Input: part model. Units: mm. Frame: model coordinates. Coordinates: 2 decimals unless noted, no trailing zeros. Write each loop counter-clockwise with the first axis right and the second up, starting at its lowest first coordinate (ties: lowest second). Pieces come first, ordered by that corner, then holes.
1) Pin query (flat end, axial travel): pin 1 Ø1.4 at (x, z) = (30, 3.5) entering from +Y; pin 2 Ø1.4 at (x, z) = (27, 1.5) entering from -Y; pin 3 Ø2 at (y, z) = (56.5, 1.5) entering from +X. Return the tip coordinate at first contact, or that it passes through.
2) Draft query along X for faces 1 (the flat face through (40.2, 62.9, 2.3)), 2 (the flat face through (53, 38, 4.572)). Return one class per face: pulls with the +X half, pulls with the -X half, needs draft (parallel to the pull), parting line crosses it, or undercut.
3) Section query C-C (z = 2.65). State how many separate pieces and enclosed holes the cut face has, then the cut area to 3 significant figures.
4) Line query: L1, parallel to Y at x = -2.5, z = 0.4 (1 decimal); L2, parallel to Y at x = 65.5, z = 3.2; L3, parallel to X at y = 42.5, z = 1. Output: solid intervals per line, ascending.
5) Section query A-A (y = 46). Output: boundary loops of the cut face in (x, z), then the cut area to 3 significant figures.
6) Section query B-B (x = 91). Output: boundary loops of the cut face in (y, z), then the cut area to 3 significant figures.
from build123d import *

# Parameters (mm, degrees)
SKETCH1_R           = 2.5527
SKETCH1_R_2         = 4.1275
SKETCH1_R_3         = 19.177
BOSS_EXTRUDE1_DEPTH = 4.572


with BuildPart() as part:
    # Sketch1 → Boss-Extrude1 (new body)
    with BuildSketch(Plane.XY):
        with BuildLine():
            Line((-17.186005785, 5.917481167), (-17.186005785, 69.562080021))
            ThreePointArc((-17.186005785, 69.562080021), (-15.770600509, 73.558612882), (-12.155368019, 75.773503633))
            Line((-12.155368019, 75.773503633), (114.857780393, 75.773503633))
            ThreePointArc((114.857780393, 75.773503633), (119.939137204, 73.478410267), (121.251078966, 68.059328295))
            Line((121.251078966, 68.059328295), (121.251078966, 4.414729441))
            ThreePointArc((121.251078966, 4.414729441), (118.772241914, 0.732566989), (114.487440215, -0.426496367))
            Line((114.487440215, -0.426496367), (-11.1125, -0.426496367))
            ThreePointArc((-11.1125, -0.426496367), (-15.422847741, 1.526196519), (-17.186005785, 5.917481167))
        make_face()
        with Locations((90.763994215, 5.917481167)):
            Circle(SKETCH1_R, mode=Mode.SUBTRACT)
        with Locations((90.763994215, 69.562080021)):
            Circle(SKETCH1_R, mode=Mode.SUBTRACT)
        with Locations((-10.836005785, 69.562080021)):
            Circle(SKETCH1_R, mode=Mode.SUBTRACT)
        with Locations((39.963994215, 69.562080021)):
            Circle(SKETCH1_R, mode=Mode.SUBTRACT)
        with Locations((-10.836005785, 5.917481167)):
            Circle(SKETCH1_R, mode=Mode.SUBTRACT)
        with Locations((39.963994215, 5.917481167)):
            Circle(SKETCH1_R, mode=Mode.SUBTRACT)
        with Locations((63.001987758, 56.151789166)):
            Circle(SKETCH1_R_2, mode=Mode.SUBTRACT)
        with Locations((115.233146458, 39.581556975)):
            Circle(SKETCH1_R, mode=Mode.SUBTRACT)
        with Locations((98.923012242, 20.230764682)):
            Circle(SKETCH1_R_2, mode=Mode.SUBTRACT)
        with Locations((80.9625, 38.1)):
            Circle(SKETCH1_R_3, mode=Mode.SUBTRACT)
        Polygon((1.103378735, 60.325), (-1.829560633, 65.405), (-7.695439367, 65.405), (-10.628378735, 60.325), (-7.695439367, 55.245), (-1.829560633, 55.245), align=None, mode=Mode.SUBTRACT)
        Polygon((50.443227049, 60.325), (47.510287682, 65.405), (41.644408947, 65.405), (38.71146958, 60.325), (41.644408947, 55.245), (47.510287682, 55.245), align=None, mode=Mode.SUBTRACT)
        Polygon((1.103378735, 16.331279268), (-1.829560633, 21.411279268), (-7.695439367, 21.411279268), (-10.628378735, 16.331279268), (-7.695439367, 11.251279268), (-1.829560633, 11.251279268), align=None, mode=Mode.SUBTRACT)
        Polygon((50.443227049, 16.331279268), (47.510287682, 21.411279268), (41.644408947, 21.411279268), (38.71146958, 16.331279268), (41.644408947, 11.251279268), (47.510287682, 11.251279268), align=None, mode=Mode.SUBTRACT)
        Polygon((68.867866493, 20.230764682), (65.934927125, 25.310764682), (60.06904839, 25.310764682), (57.136109023, 20.230764682), (60.06904839, 15.150764682), (65.934927125, 15.150764682), align=None, mode=Mode.SUBTRACT)
        Polygon((104.788890977, 56.151789166), (101.85595161, 61.231789166), (95.990072875, 61.231789166), (93.057133507, 56.151789166), (95.990072875, 51.071789166), (101.85595161, 51.071789166), align=None, mode=Mode.SUBTRACT)
        Polygon((24.915878735, 47.625), (21.982939367, 52.705), (16.117060633, 52.705), (13.184121265, 47.625), (16.117060633, 42.545), (21.982939367, 42.545), align=None, mode=Mode.SUBTRACT)
        Polygon((34.440878735, 38.1), (31.507939367, 43.18), (25.642060633, 43.18), (22.709121265, 38.1), (25.642060633, 33.02), (31.507939367, 33.02), align=None, mode=Mode.SUBTRACT)
    extrude(amount=BOSS_EXTRUDE1_DEPTH)


solid = part.part
Answer:
1. pin 1: stops at y = 75.77
1. pin 2: stops at y = -0.43
1. pin 3: stops at x = 121.25
2. face 1: undercut
2. face 2: needs draft
3. separate pieces: 1
3. enclosed holes: 18
3. area: 8,400 mm2
4. L1: y = -0.4 to 11.3, 21.4 to 55.2, 65.4 to 75.8
4. L2: y = -0.43 to 15.15, 25.31 to 26.76, 49.44 to 52.87, 59.44 to 75.77
4. L3: x = -17.19 to 25.25, 31.9 to 62.3, 99.63 to 121.25
5. outline: (-17.19, 0) - (14.12, 0) - (14.12, 4.57) - (-17.19, 4.57) - close; (23.98, 0) - (63.49, 0) - (63.49, 4.57) - (23.98, 4.57) - close; (98.44, 0) - (121.25, 0) - (121.25, 4.57) - (98.44, 4.57) - close
5. area: 428 mm2
6. outline: (-0.43, 0) - (3.38, 0) - (3.38, 4.57) - (-0.43, 4.57) - close; (8.46, 0) - (21.76, 0) - (21.76, 4.57) - (8.46, 4.57) - close; (54.44, 0) - (67.02, 0) - (67.02, 4.57) - (54.44, 4.57) - close; (72.1, 0) - (75.77, 0) - (75.77, 4.57) - (72.1, 4.57) - close
6. area: 152 mm2
